Part model, mm, in its own coordinate system. A direction names the side the tool comes from. Give positions to 0.01 mm unless a question says otherwise; leave off trailing zeros. Order: outer loops, then holes, each group sorted by start corner. A loop starts at its lowest first (then second) coordinate and runs counter-clockwise, first axis right, second up. Notation, with made-up numbers: (3.25, 79) - (23.25, 79) arc R32 cw to (23.25, 115) - close; hole circle Ø3 at (-11, 0.25). An arc over 180 degrees is marked (long way). One line per item, written item: value.
```python
from build123d import *


with BuildPart() as f1:
    # F0 (on Front) → F1 (revolve)
    with BuildSketch(Plane.XZ):
        with BuildLine():
            Line((-39.205529, 93.758564), (-40, 93.151263))
            Line((-40, 93.151263), (-3, 44.747897))
            Line((-3, 44.747897), (-3, -17.268907))
            ThreePointArc((-3, -17.268907), (-15.880826, -23.803916), (-30, -26.848737))
            Line((-30, -26.848737), (-29.916253, -27.845224))
            ThreePointArc((-29.916253, -27.845224), (-15.296707, -24.657094), (-2, -17.794671))
            Line((-2, -17.794671), (-2, 45.086327))
            Line((-2, 45.086327), (-39.205529, 93.758564))
        make_face()
    revolve(axis=Axis((0, 0, 33.025213), (0, 0, -1)))


solid = f1.part
```
1) Cut at A-A, the plane z = 24. Give the cut face in (x, y).
Outcome:
outline: circle Ø6 at (0, 0); hole circle Ø4 at (0, 0)
2) Pin check, flat tips, straight feed: pin 1 (2.5 mm diameter, centred on x = 0, y = 0, fed in from +Z); pin 2 (1 mm diameter, centred on x = 2, z = -4.5, fed in from +Y); pin 3 (1 mm diameter, centred on x = 9.5, y = -8.5, fed in from +Z). Stop position of each tip, or through.
Outcome:
pin 1: passes through
pin 2: stops at y = 2.6
pin 3: stops at z = 59.8
3) Drill centre lines: line 1 along Y through (x, z) = (0, -1); line 2 along Z through (x, y) = (21, 17.5); line 3 along Z through (x, y) = (-22.5, -8). Where is each one in solid material? Low to high. Write a range as from..to.
Outcome:
line 1: y = -3..-2, 2..3
line 2: z = -27.57..-26.56, 76.58..78.23
line 3: z = -27.01..-25.99, 72.06..73.71
4) Which spindle directions (+Z, -Z, +X, -X, +Y, -Y) get a long thin tool onto all of the face, cutting with end or side? Do faces 1 (the conical face through (10.33, -7.92, 57.85)), 2 (the cylindrical face through (0, -2, 14)). Say none if no direction does.
Outcome:
face 1: none
face 2: +Z, -Z
5) Mould opens along Y. For faces 3 (the cylindrical face through (3, 0, 13)), 4 (the conical face through (-12.014, 3.783, 58.947)) say: released by +Y, released by -Y, zero draft, split by the parting line, or undercut.
Outcome:
face 3: split by the parting line
face 4: undercut
